```python
from build123d import *

# Parameters (mm, degrees)
F1_DEPTH    = 74.93201
F2_T1_DEPTH = 161.3731420762
F2_T3_DEPTH = 161.3731420762
F2_T5_DEPTH = 161.3731420762
F2_T7_DEPTH = 161.3731420762


# Not quite as in the source:
# - a fillet or chamfer that OpenCascade refuses, or shapes differently, is made with other operations: its cross-section is extruded or revolved along the edge and cut away or added


with BuildPart() as f1:
    # F0 (on Top) → F1 (new body)
    with BuildSketch(Plane.XY):
        Polygon((-56.1133213341, -3.1524337828), (-31.7345000803, 53.1710572541), (-88.0579911172, 77.5498785079), (-112.436812371, 21.226387471), align=None)
    extrude(amount=F1_DEPTH)

    # F2: fillet of radius 20 on 4 edges, made by hand

    # F2_s2 → F2_t1 (cut)
    with BuildSketch(Plane(origin=(-29.8642383226, -68.9966976654, 0), x_dir=(0, 0, 1), z_dir=(0.3972229615, 0.917722136, 0))):
        with BuildLine():
            add(Edge.make_bspline(
                [(54.93201, -50.2442180275), (74.93201, -50.2442180275), (74.93201, -70.2442180275)],
                knots=[0, 0, 0, 1, 1, 1], degree=2, weights=[1, 1, 1]))
            Line((74.93201, -70.2442180275), (74.93201, -50.2442180275))
            Line((74.93201, -50.2442180275), (54.93201, -50.2442180275))
        make_face()
    extrude(amount=F2_T1_DEPTH, mode=Mode.SUBTRACT)

    # F2_s4 → F2_t3 (cut)
    with BuildSketch(Plane(origin=(-0.2241242898, 0.0970090081, 0), x_dir=(0, 0, 1), z_dir=(-0.917722136, 0.3972229615, 0))):
        with BuildLine():
            add(Edge.make_bspline(
                [(54.93201, 36.1905841301), (74.93201, 36.1905841301), (74.93201, 16.1905841301)],
                knots=[0, 0, 0, 1, 1, 1], degree=2, weights=[1, 1, 1]))
            Line((74.93201, 16.1905841301), (74.93201, 36.1905841301))
            Line((74.93201, 36.1905841301), (54.93201, 36.1905841301))
        make_face()
    extrude(amount=F2_T3_DEPTH, mode=Mode.SUBTRACT)

    # F2_s6 → F2_t5 (cut)
    with BuildSketch(Plane(origin=(34.236879084, 79.0990069677, 0), x_dir=(0, 0, 1), z_dir=(-0.3972229615, -0.917722136, 0))):
        with BuildLine():
            add(Edge.make_bspline(
                [(54.93201, 111.6173601037), (74.93201, 111.6173601037), (74.93201, 91.6173601037)],
                knots=[0, 0, 0, 1, 1, 1], degree=2, weights=[1, 1, 1]))
            Line((74.93201, 91.6173601037), (74.93201, 111.6173601037))
            Line((74.93201, 111.6173601037), (54.93201, 111.6173601037))
        make_face()
    extrude(amount=F2_T5_DEPTH, mode=Mode.SUBTRACT)

    # F2_s8 → F2_t7 (cut)
    with BuildSketch(Plane(origin=(-148.3198289229, 64.1981264147, 0), x_dir=(0, 0, 1), z_dir=(0.917722136, -0.3972229615, 0))):
        with BuildLine():
            add(Edge.make_bspline(
                [(54.93201, 25.1825579461), (74.93201, 25.1825579461), (74.93201, 5.1825579461)],
                knots=[0, 0, 0, 1, 1, 1], degree=2, weights=[1, 1, 1]))
            Line((74.93201, 5.1825579461), (74.93201, 25.1825579461))
            Line((74.93201, 25.1825579461), (54.93201, 25.1825579461))
        make_face()
    extrude(amount=F2_T7_DEPTH, mode=Mode.SUBTRACT)


solid = f1.part
```
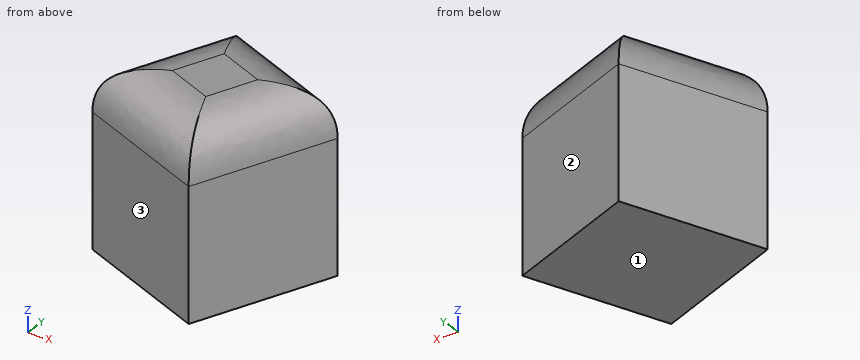
Geometry check sheet. Reference: the model listing, model coordinates, mm. Face numbers are marked on the shaded views. Coordinates: 2 decimals unless noted, no trailing zeros. Order: outer loops, then holes, each group sorted by start corner. A loop starts at its lowest first (then second) coordinate and runs counter-clockwise, first axis right, second up. Notation, with made-up numbers: (-24, -17.5) - (3, -17.5) arc R34 cw to (3, 21.5) - close; hole circle Ø10 at (63, 78). An arc over 180 degrees is marked (long way). Use one line per item in the form item = value.
1. Section check A-A (z = 18). Record the boundary of the cut face in (x, y).
Here are the results:
outline = (-112.44, 21.23) - (-56.11, -3.15) - (-31.73, 53.17) - (-88.06, 77.55) - close
2. Draft check along X on the marked faces 1, 2 and 3. Enter one of: pulls with the +X half, pulls with the -X half, needs draft (parallel to the pull), parting line crosses it, or undercut.
Here are the results:
face_1 = needs draft
face_2 = pulls with the +X half
face_3 = pulls with the -X half
3. Scan lines: line 1 (Y direction, x = -84, z = 35); line 2 (X direction, y = 37, z = 29.5); line 3 (X direction, y = 16, z = 12). Record each from-to range of solid material in increasing order.
Here are the results:
line_1 = 8.92 to 75.79
line_2 = -105.61 to -38.73
line_3 = -100.36 to -47.82
4. Gauge pin test, flat ends, axial feed: pin 1 (2 mm diameter, centred on y = 39, z = 60.5, fed in from -X); pin 2 (5 mm diameter, centred on x = -47, z = 21, fed in from +Y); pin 3 (8 mm diameter, centred on x = -61, y = 8.5, fed in from +Z); pin 4 (12 mm diameter, centred on x = -41, y = 14, fed in from +Z). Record the tip position at first contact, or that the pin passes through.
Here are the results:
pin_1 = -104.72
pin_2 = 60.86
pin_3 = 73.84
pin_4 = through
